CAD build for the part. Positions are in the model's coordinates, mm. Face numbers are marked on the shaded views. A direction names the side the tool comes from. Round coordinates to 2 decimals unless told otherwise and drop trailing zeros. Loops run counter-clockwise (first coordinate to the right, second up) from the corner with the lowest first, then second, coordinate; pieces in that order, holes last. Notation, with made-up numbers: M 73.5,39 L 128.5,39 A17 ccw 128.5,63 Z; hole C 6.5,-38 d3. An arc over 180 degrees is marked long. Use a Markdown table: item, result. Add a question column.
(1) Band-saw the part on D-D, the plane y = 4.5. Write the cut outline in (x, z), and give its area (3 significant figures).
(2) Two-plate mould, pull along Y, no slides. Class the marked faces 6, 7, 8 and 9: released by +Y, released by -Y, zero draft, split by the parting line, or undercut.
(3) Which spindle directions (+Z, -Z, +X, -X, +Y, -Y) get a long thin tool onto all of the face, cutting with end or side? Do the marked faces 1, 2, 3, 4 and 5. Say none if no direction does.
(4) Wall check: L1, parallel to X at y = 3.5, z = -3.5; L2, parallel to X at y = 6.5, z = 0.5; L3, parallel to X at y = 4.75, z = 1.5. Give the ranges that are in metal, low to high.
(5) Band-saw the part on A-A, the plane x = 0. Write the cut outline in (y, z).
(6) Band-saw the part on B-B, the plane z = 0.25. Write the cut outline in (x, y), and give its area (3 significant figures).
(7) Flat gauge pins, fed straight in: P1, Ø1, axis at y = 6, z = 2, coming from the +X side; P2, Ø3.5, axis at y = 3, z = -1.5, coming from the +X side; P3, Ø1, axis at x = -2.5, z = 2.5, coming from the +Y side; P4, Ø2, axis at x = 4.5, z = 0.5, coming from the +Y side. Where does each tip first touch, or does it go through?
(8) Band-saw the part on C-C, the plane y = 3. Write the cut outline in (x, z).
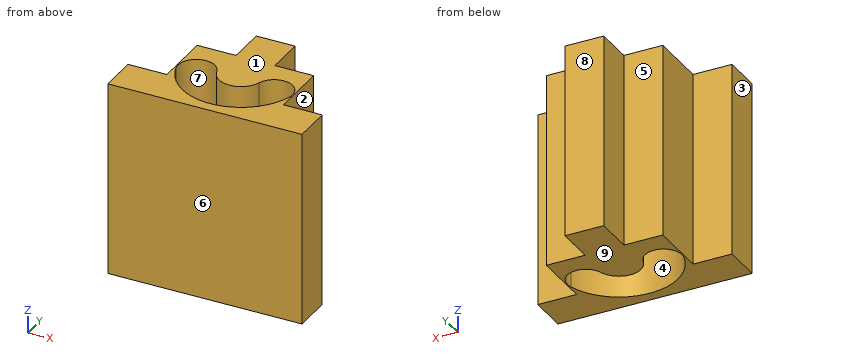
from build123d import *

# Parameters (mm, degrees)
BOSS_EXTRUDE1_DEPTH = 5
CUT_EXTRUDE1_DEPTH  = 10


with BuildPart() as part:
    # Sketch1 → Boss-Extrude1 (new, symmetric)
    with BuildSketch(Plane.XY):
        Polygon((-5, 0), (5, 0), (5, 2), (3, 2), (3, 5), (1, 5), (1, 7), (-1, 7), (-1, 5), (-3, 5), (-3, 2), (-5, 2), align=None)
    extrude(amount=BOSS_EXTRUDE1_DEPTH, both=True)

    # Sketch2 → Cut-Extrude1 (cut)
    with BuildSketch(Plane.XY.offset(5)):
        with BuildLine():
            ThreePointArc((-2.911371351, 2.73185403), (0, 0.553674644), (2.911371351, 2.73185403))
            ThreePointArc((2.911371351, 2.73185403), (2.26814597, 3.911371351), (1.088628649, 3.26814597))
            ThreePointArc((1.088628649, 3.26814597), (0, 2.453674644), (-1.088628649, 3.26814597))
            ThreePointArc((-1.088628649, 3.26814597), (-2.26814597, 3.911371351), (-2.911371351, 2.73185403))
        make_face()
    extrude(amount=-CUT_EXTRUDE1_DEPTH, mode=Mode.SUBTRACT)


solid = part.part
Return value:
| question | item | result |
|---|---|---|
| 1 | outline | M -3,-5 L 3,-5 L 3,5 L -3,5 Z |
| 1 | area | 60.0 mm^2 |
| 2 | face 6 | released by -Y |
| 2 | face 7 | undercut |
| 2 | face 8 | released by +Y |
| 2 | face 9 | zero draft |
| 3 | face 1 | +Z, +X, -X, +Y, -Y |
| 3 | face 2 | +Z, -Z, +X, +Y |
| 3 | face 3 | +Z, -Z, -X, +Y, -Y |
| 3 | face 4 | +Z, -Z |
| 3 | face 5 | +Z, -Z, -X, +Y |
| 4 | L1 | -3 to -2.81, -1.19 to 1.19, 2.81 to 3 |
| 4 | L2 | -1 to 1 |
| 4 | L3 | -3 to 3 |
| 5 | outline | M 0,-5 L 0.55,-5 L 0.55,5 L 0,5 Z; M 2.45,-5 L 7,-5 L 7,5 L 2.45,5 Z |
| 6 | outline | M -5,0 L 5,0 L 5,2 L 3,2 L 3,5 L 1,5 L 1,7 L -1,7 L -1,5 L -3,5 L -3,2 L -5,2 Z; hole M -2.91,2.73 A3.03 ccw 2.91,2.73 A0.95 ccw 1.09,3.27 A1.13 cw -1.09,3.27 A0.95 ccw Z |
| 6 | area | 29.0 mm^2 |
| 7 | P1 | x = 1 |
| 7 | P2 | x = 5 |
| 7 | P3 | y = 5 |
| 7 | P4 | y = 2 |
| 8 | outline | M -3,-5 L -2.95,-5 L -2.95,5 L -3,5 Z; M -0.97,-5 L 0.97,-5 L 0.97,5 L -0.97,5 Z; M 2.95,-5 L 3,-5 L 3,5 L 2.95,5 Z |
